```python
from build123d import *

# Parameters (mm, degrees)
BOSS_EXTRUDE1_DEPTH = 5
SKETCH2_W           = 9.2
SKETCH2_H           = 5.5
BOSS_EXTRUDE2_DEPTH = 1
CHAMFER1_SIZE       = 0.6


with BuildPart() as part:
    # Sketch1 → Boss-Extrude1 (new body)
    with BuildSketch(Plane.XY):
        with BuildLine():
            Line((-4.17, -0.3), (-1.3, -0.3))
            ThreePointArc((-1.3, -0.3), (-0.592893219, -0.592893219), (-0.3, -1.3))
            Line((-0.3, -1.3), (-0.3, -1.86))
            ThreePointArc((-0.3, -1.86), (-0.592893219, -2.567106781), (-1.3, -2.86))
            Line((-1.3, -2.86), (-7.65, -2.86))
            ThreePointArc((-7.65, -2.86), (-8.357106781, -2.567106781), (-8.65, -1.86))
            Line((-8.65, -1.86), (-8.65, -1.3))
            ThreePointArc((-8.65, -1.3), (-8.357106781, -0.592893219), (-7.65, -0.3))
            Line((-7.65, -0.3), (-4.17, -0.3))
        make_face()
    extrude(amount=BOSS_EXTRUDE1_DEPTH)

    # Sketch2 → Boss-Extrude2 (add)
    with BuildSketch(Plane.XY.offset(5)):
        with Locations((-4.475, -2.81)):
            Rectangle(SKETCH2_W, SKETCH2_H)
    extrude(amount=-BOSS_EXTRUDE2_DEPTH)

    # Chamfer1
    chamfer1_edges = [part.edges().sort_by_distance(p)[0] for p in [
        (0.125, -0.06, 4.5),
        (0.125, -5.56, 4.5),
        (-9.075, -5.56, 4.5),
        (-9.075, -0.06, 4.5),
    ]]
    chamfer(chamfer1_edges, length=CHAMFER1_SIZE)


solid = part.part
```
For this review, take the finished solid that the model builds, in its own axes (mm). A direction names the side the tool comes from. Round coordinates to 2 decimals unless told otherwise and drop trailing zeros. Order: outer loops, then holes, each group sorted by start corner. A loop starts at its lowest first (then second) coordinate and runs counter-clockwise, first axis right, second up. Notation, with made-up numbers: (3.5, 30) -> (12.5, 30) arc R13 cw to (12.5, 37) -> close; hole circle Ø1 at (44, -29). An arc over 180 degrees is marked (long way). Use a Markdown table: item, result.
Item 1: For pin 1 (2 mm diameter, centred on x = -7, z = 1, fed in from +Y); pin 2 (1.5 mm diameter, centred on y = -2, z = 2, fed in from -X); pin 3 (3 mm diameter, centred on x = -5, z = 1.5, fed in from -Y), all flat-tipped, find the tip position at first contact; note any pin that passes through.
Resolved:
| item | result |
|---|---|
| pin 1 | stops at y = -0.3 |
| pin 2 | stops at x = -8.65 |
| pin 3 | stops at y = -2.86 |
Item 2: Take a section at A-A (x = -3). State the section outline as (y, z) points.
Resolved:
| item | result |
|---|---|
| outline | (-5.56, 4) -> (-2.86, 4) -> (-2.86, 0) -> (-0.3, 0) -> (-0.3, 4) -> (-0.06, 4) -> (-0.06, 5) -> (-5.56, 5) -> close |
Item 3: Take a section at B-B (z = 3.75). State the section outline as (x, y) points.
Resolved:
| item | result |
|---|---|
| outline | (-8.65, -1.86) arc R1 ccw to (-7.65, -2.86) -> (-1.3, -2.86) arc R1 ccw to (-0.3, -1.86) -> (-0.3, -1.3) arc R1 ccw to (-1.3, -0.3) -> (-7.65, -0.3) arc R1 ccw to (-8.65, -1.3) -> close |
Item 4: Machinability: for faces 1 (the cylindrical face through (-0.585, -2.559, 1.972)), 2 (the cylindrical face through (-0.601, -0.585, 1.972)), 3 (the flat face through (-5, -0.3, 2)), 4 (the cylindrical face through (-8.365, -0.601, 1.972)), 5 (the flat face through (-4, -2.86, 2)), which of the approach directions +Z, -Z, +X, -X, +Y, -Y give a long, thin tool a straight path to every point of the face, cutting with its end or side? Answer none if there is none.
Resolved:
| item | result |
|---|---|
| face 1 | -Z, +X, -Y |
| face 2 | -Z, +X, +Y |
| face 3 | -Z, +X, -X, +Y |
| face 4 | -Z, -X, +Y |
| face 5 | -Z, +X, -X, -Y |
Item 5: Take a section at C-C (y = -4.5). State the section outline as (x, z) points (3 decimals).
Resolved:
| item | result |
|---|---|
| outline | (-9.075, 4) -> (0.125, 4) -> (0.125, 5) -> (-9.075, 5) -> close |
Item 6: For line 1 along Z through (x, y) = (-3, -3.55); line 2 along Y through (x, z) = (-3, 2); line 3 along X through (y, z) = (-1.25, 2), list the stretches that pass through material, from the lowest coordinate up. Write a range as [from, to].
Resolved:
| item | result |
|---|---|
| line 1 | z = [4, 5] |
| line 2 | y = [-2.86, -0.3] |
| line 3 | x = [-8.65, -0.3] |
